```python
from build123d import *

# Parameters (mm, degrees)
CYLINDER015_R                      = 2.5
CYLINDER015_DEPTH                  = 23
CYLINDER014_R                      = 4.36
CYLINDER014_DEPTH                  = 5
FUSION001018017018_PLACEMENT_ANGLE = 180
POCKET002018004_DEPTH              = 2.5


with BuildPart() as cylinder015:
    # Cylinder015 → Cylinder015 (new body)
    with BuildSketch(Plane.XY):
        Circle(CYLINDER015_R)
    extrude(amount=CYLINDER015_DEPTH)


with BuildPart() as obj1:
    # Cylinder014 → Cylinder014 (new body)
    with BuildSketch(Plane.XY):
        Circle(CYLINDER014_R)
    extrude(amount=CYLINDER014_DEPTH)

    # Fusion001018017018: union Cylinder015
    add(cylinder015.part)


with BuildPart() as obj1_1:
    # Fusion001018017018 placement: moved
    add(obj1.part.rotate(Axis((0, 0, 0), (0, 1, 0)), FUSION001018017018_PLACEMENT_ANGLE))

    # Sketch020 → Pocket002018004 (cut)
    with BuildSketch(Plane(origin=(0, 0, 0), x_dir=(-1, 0, 0), z_dir=(0, 0, 1))):
        Polygon((2, -1.154701), (2, 1.154701), (0, 2.309401), (-2, 1.154701), (-2, -1.154701), (0, -2.309401), align=None)
    extrude(amount=-POCKET002018004_DEPTH, mode=Mode.SUBTRACT)


solid = obj1_1.part
```
CAD build for the part. Positions are in the model's coordinates, mm. A direction names the side the tool comes from. Round coordinates to 2 decimals unless told otherwise and drop trailing zeros. Order: outer loops, then holes, each group sorted by start corner. A loop starts at its lowest first (then second) coordinate and runs counter-clockwise, first axis right, second up. Notation, with made-up numbers: (17, 64) - (44, 64) arc R31 ccw to (44, 101) - close; hole circle Ø10 at (19, 70). An arc over 180 degrees is marked (long way). Answer in a Markdown table with one row per item. Add a question column.
(1) Band-saw the part on C-C on x = 1. List the corners of the cut face in (y, z).
(2) Band-saw the part on A-A on y = 0. List the corners of the cut face in (x, z), and give its area (3 significant figures).
(3) Band-saw the part on B-B on z = -4.25. List the corners of the cut face in (x, y), and give its area (3 significant figures).
(4) Band-saw the part on D-D on z = -21.25. List the corners of the cut face in (x, y), and give its area (3 significant figures).
(5) 3-axis set-ups, long thin cutter, end or side, ignore diameter. For faces 5 (the face through (0, 0, -23)), 6 (the face through (-2, -2, -5)), 7 (the face through (0, 0, -2.5)): which of +Z, -Z, +X, -X, +Y, -Y reach the whole face in a straight line?
(6) Drop flat-ended pins along their axis: pin 1 Ø1.5 at (x, z) = (1.5, -14.5) entering from +Y; pin 2 Ø3 at (x, z) = (1.5, -9.5) entering from +Y; pin 3 Ø1.5 at (x, z) = (-1, -2.5) entering from +Y. Give the stop position or say it passes through.
(7) Mould opens along X. For faces 1 (the face through (-2, 0, -1)), 2 (the face through (2, 0, -1)), 3 (the face through (-1, -2, 0)), 4 (the face through (0.54, -2.44, -13.87)) say: +X half, -X half, draft (parallel to the pull), parting line (faces both ways), or undercut.
(8) Probe L1, parallel to Z at x = 0.25, y = 0.5; L2, parallel to Z at x = 3, y = 0.25; L3, parallel to X at y = 2.25, z = -2.25. List the from-to ranges inside material, lowest first. Write a range as [from, to].
Data:
| question | item | result |
|---|---|---|
| 1 | outline | (-4.24, -5) - (-2.29, -5) - (-2.29, -23) - (2.29, -23) - (2.29, -5) - (4.24, -5) - (4.24, 0) - (1.73, 0) - (1.73, -2.5) - (-1.73, -2.5) - (-1.73, 0) - (-4.24, 0) - close |
| 2 | outline | (-4.36, -5) - (-2.5, -5) - (-2.5, -23) - (2.5, -23) - (2.5, -5) - (4.36, -5) - (4.36, 0) - (2, 0) - (2, -2.5) - (-2, -2.5) - (-2, 0) - (-4.36, 0) - close |
| 2 | area | 124 mm^2 |
| 3 | outline | circle Ø8.72 at (0, 0) |
| 3 | area | 59.7 mm^2 |
| 4 | outline | circle Ø5 at (0, 0) |
| 4 | area | 19.6 mm^2 |
| 5 | face 5 | -Z, +X, -X, +Y, -Y |
| 5 | face 6 | -Z |
| 5 | face 7 | +Z |
| 6 | pin 1 | stops at y = 2.38 |
| 6 | pin 2 | stops at y = 2.5 |
| 6 | pin 3 | stops at y = 4.35 |
| 7 | face 1 | undercut |
| 7 | face 2 | undercut |
| 7 | face 3 | draft |
| 7 | face 4 | parting line |
| 8 | L1 | z = [-23, -2.5] |
| 8 | L2 | z = [-5, 0] |
| 8 | L3 | x = [-3.73, -0.1], [0.1, 3.73] |
